Geometry: final body of the model. Coordinates: model frame, mm. A direction names the side the tool comes from. Give positions to 0.01 mm unless a question says otherwise; leave off trailing zeros. Order: outer loops, then holes, each group sorted by start corner. A loop starts at its lowest first (then second) coordinate and runs counter-clockwise, first axis right, second up. Notation, with made-up numbers: M 62,52.25 L 95,52.25 A28 ccw 95,72.25 Z; hole C 49,-21 d5. An arc over 180 degrees is marked long. Write item = value, one per line. Start each with the question number.
from build123d import *

# Parameters (mm, degrees)
SKETCH1_W      = 74.93
SKETCH1_H      = 59.436
EXTRUDE1_DEPTH = 1.5875
SKETCH2_W      = 62.23
SKETCH2_H      = 46.736
EXTRUDE2_DEPTH = 1.5875


with BuildPart() as part:
    # Sketch1 → Extrude1 (new body)
    with BuildSketch(Plane.XY):
        with Locations((37.465, 29.718)):
            Rectangle(SKETCH1_W, SKETCH1_H)
    extrude(amount=-EXTRUDE1_DEPTH)

    # Sketch2 → Extrude2 (add)
    with BuildSketch(Plane.XY):
        with Locations((37.465, 29.718)):
            Rectangle(SKETCH2_W, SKETCH2_H)
    extrude(amount=EXTRUDE2_DEPTH)


solid = part.part
1) Cut plane B-B (x = 23.5). Return loops of the section in (y, z), plus the area to 3 significant figures.
2) Ray query, L1, parallel to Y at x = 10, z = 0.05; L2, parallel to X at y = 35, z = 0.45; L3, parallel to Z at x = 17, y = 53.5. Return the intervals inside material, ascending.
3) Cut plane C-C (z = 0.85). Return loops of the section in (x, y), plus the area to 3 significant figures.
4) Cut plane A-A (y = 9). Return loops of the section in (x, z).
5) Pin query (flat end, axial travel): pin 1 Ø1 at (y, z) = (29.5, -1) entering from -X; pin 2 Ø0.8 at (x, z) = (39.5, 0.5) entering from -Y; pin 3 Ø0.8 at (y, z) = (34, 1) entering from -X; pin 4 Ø0.5 at (x, z) = (34.5, 1) entering from +Y. Return the tip coordinate at first contact, or that it passes through.
6) Access query for faces 1 (the flat face through (37, 6.35, 1)), 2 (the flat face through (74.93, 29, -1)), 3 (the flat face through (68.58, 29, 1)), 4 (the flat face through (6.35, 29, 1)), 5 (the flat face through (37, 53.086, 1)). Directions: +Z, -Z, +X, -X, +Y, -Y. A direction counts if a zero-diameter tool reaches every point of the face in a straight line with its end or side. Return the directions, or none.
7) Cut plane D-D (x = 5). Return loops of the section in (y, z), plus the area to 3 significant figures.
Reply:
q1.outline = M 0,-1.59 L 59.44,-1.59 L 59.44,0 L 53.09,0 L 53.09,1.59 L 6.35,1.59 L 6.35,0 L 0,0 Z
q1.area = 169 mm²
q2.L1 = 6.35 to 53.09
q2.L2 = 6.35 to 68.58
q2.L3 = -1.59 to 0
q3.outline = M 6.35,6.35 L 68.58,6.35 L 68.58,53.09 L 6.35,53.09 Z
q3.area = 2,910 mm²
q4.outline = M 0,-1.59 L 74.93,-1.59 L 74.93,0 L 68.58,0 L 68.58,1.59 L 6.35,1.59 L 6.35,0 L 0,0 Z
q5.pin_1 = 0
q5.pin_2 = 6.35
q5.pin_3 = 6.35
q5.pin_4 = 53.09
q6.face_1 = +Z, +X, -X, -Y
q6.face_2 = +Z, -Z, +X, +Y, -Y
q6.face_3 = +Z, +X, +Y, -Y
q6.face_4 = +Z, -X, +Y, -Y
q6.face_5 = +Z, +X, -X, +Y
q7.outline = M 0,-1.59 L 59.44,-1.59 L 59.44,0 L 0,0 Z
q7.area = 94.4 mm²
